from build123d import *

# Parameters (mm, degrees)
F0_R     = 4.7625
F0_R_2   = 2.3876
F1_DEPTH = 6.35
F3_DEPTH = 6.351
F4_R     = 0.254


with BuildPart() as f1:
    # F0 (on Front) → F1 (new body)
    with BuildSketch(Plane.XZ):
        Circle(F0_R)
        Circle(F0_R_2, mode=Mode.SUBTRACT)
    extrude(amount=F1_DEPTH)

    # F2 (on face) → F3 (cut, through all)
    with BuildSketch(Plane.XZ.offset(6.35)):
        Polygon((-2.794, -1.778), (-4.8590770571, 3.8957525837), (-7.3392285321, 3.8957525837), (-7.3392285321, -6.9893564564), (6.3704967257, -6.9893564564), (6.3704967257, 4.2867070974), (5.001372863, 4.2867070974), (2.794, -1.778), align=None)
    extrude(amount=-F3_DEPTH, mode=Mode.SUBTRACT)

    # F4
    f4_edges = [f1.edges().sort_by_distance(p)[0] for p in [
        (-1.593534, -3.175, -1.778),
        (1.593534, -3.175, -1.778),
    ]]
    fillet(f4_edges, radius=F4_R)


solid = f1.part
Geometry check sheet. Reference: the model listing, model coordinates, mm. Give positions to 0.01 mm unless a question says otherwise; leave off trailing zeros. Order: outer loops, then holes, each group sorted by start corner. A loop starts at its lowest first (then second) coordinate and runs counter-clockwise, first axis right, second up. Notation, with made-up numbers: M 46,-11.5 L 83,-11.5 A25 ccw 83,12.5 Z; hole C 71,7 d10. An arc over 180 degrees is marked long. Use a Markdown table: item, result.
Item 1: Section check C-C (x = 0). Record the cut outline in (y, z).
Answers follow:
| item | result |
|---|---|
| outline | M -6.35,2.39 L 0,2.39 L 0,4.76 L -6.35,4.76 Z |
Item 2: Section check A-A (z = 0). Record the cut outline in (x, y).
Answers follow:
| item | result |
|---|---|
| outline | M -3.44,-6.35 L -2.39,-6.35 L -2.39,0 L -3.44,0 Z; M 2.39,-6.35 L 3.44,-6.35 L 3.44,0 L 2.39,0 Z |
Item 3: Material ranges on line 1 along X through (y, z) = (-1.75, 0); line 2 along X through (y, z) = (-4.5, -0.5); line 3 along Z through (x, y) = (0, -2), recorded low to high.
Answers follow:
| item | result |
|---|---|
| line 1 | x = -3.44 to -2.39, 2.39 to 3.44 |
| line 2 | x = -3.26 to -2.33, 2.33 to 3.26 |
| line 3 | z = 2.39 to 4.76 |
Item 4: Section check D-D (x = -3.25). Record the cut outline in (y, z).
Answers follow:
| item | result |
|---|---|
| outline | M -6.35,-0.53 L 0,-0.53 L 0,3.48 L -6.35,3.48 Z |
Item 5: Section check B-B (y = -3.75). Record the cut outline in (x, z) (1 decimal), and give its area (3 significant figures).
Answers follow:
| item | result |
|---|---|
| outline | M -4.2,2.2 L -2.8,-1.8 L -2.2,-1.8 A0.3 ccw -2,-1.4 A2.4 cw long 2,-1.4 A0.3 ccw 2.2,-1.8 L 2.8,-1.8 L 4.2,2.2 A4.8 ccw Z |
| area | 26.7 mm2 |
Item 6: Draft check along X on faces 1 (the flat face through (-3.504, -3.219, 0.173)), 2 (the cylindrical face through (0.073, -3.131, 2.386)), 3 (the flat face through (3.524, -3.219, 0.229)). Enter one of: +X half, -X half, draft (parallel to the pull), parting line (faces both ways), or undercut.
Answers follow:
| item | result |
|---|---|
| face 1 | -X half |
| face 2 | undercut |
| face 3 | +X half |
Item 7: Depth check by flat-ended pin: P1, Ø1, axis at y = -5, z = 1, coming from the -X side; P2, Ø3, axis at x = 0, z = 0, coming from the +Y side; P3, Ø1.5, axis at y = -3.5, z = 1, coming from the +X side. Enter the tip coordinate at first touch or a pass-through.
Answers follow:
| item | result |
|---|---|
| P1 | stops at x = -3.99 |
| P2 | passes through |
| P3 | stops at x = 4.08 |
